from build123d import *

# Parameters (mm, degrees)
F2_R     = 5
F2_R_2   = 1.5
F3_DEPTH = 7.001
F4_D     = 2.5
F4_DEPTH = 3.2
F4_TIP   = 0.7510757738
F2_R_3   = 1.2
F5_DEPTH = 3.2


with BuildPart() as f1:
    # F0 (on Front) → F1 (revolve)
    with BuildSketch(Plane.XZ):
        Polygon((8.25, 7), (0, 7), (0, 0), (8.25, 0), (8.25, 0.9163741209), (7.85, 0.9163741209), (7.85, 1.9445925065), (8.25, 1.9445925065), (8.25, 3.9838924357), (7.85, 3.9838924357), (7.85, 5.2177544985), (8.25, 5.2177544985), align=None)
    revolve(axis=Axis((0, 0, 3.5), (0, 0, 1)))

    # F2 (on Top) → F3 (cut, through all)
    with BuildSketch(Plane.XY):
        with Locations((2.75, 0)):
            Circle(F2_R)
        with Locations((-4.75, 0)):
            Circle(F2_R_2)
    extrude(amount=F3_DEPTH, mode=Mode.SUBTRACT)

    # F4
    with Locations(Plane(origin=(0, 0, 0), x_dir=(1, 0, 0), z_dir=(0, 0, -1))):
        with Locations((0, 5.75), (0, -5.75)):
            Hole(F4_D / 2, depth=F4_DEPTH)
            with Locations((0, 0, -(F4_DEPTH + F4_TIP / 2))):  # 118° drill point
                Cone(0, F4_D / 2, F4_TIP, mode=Mode.SUBTRACT)

    # F2 (on Top) → F5 (cut)
    with BuildSketch(Plane.XY):
        with Locations((0, 5.75)):
            Circle(F2_R_3)
        with Locations((0, -5.75)):
            Circle(F2_R_3)
    extrude(amount=F5_DEPTH, mode=Mode.SUBTRACT)


solid = f1.part
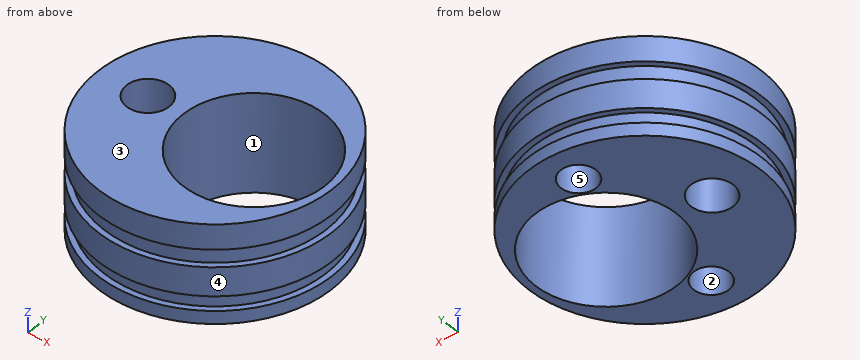
Source: CAD feature listing. Evaluate the final solid. Frame: model axes, mm. Face numbers are marked on the shaded views. A direction names the side the tool comes from. Give positions to 0.01 mm unless a question says otherwise; leave off trailing zeros. Write each loop counter-clockwise with the first axis right and the second up, starting at its lowest first coordinate (ties: lowest second). Pieces come first, ordered by that corner, then holes. Notation, with made-up numbers: M 78.5,72 L 114.5,72 A32 ccw 114.5,102 Z; hole C 60,-4.5 d2. An arc over 180 degrees is marked long. Return JSON: item names as keys, results as strings. Group by question number.
1) Set-up query: the marked faces 1 and 2. Return all of +Z, -Z, +X, -X, +Y, -Y with unobstructed straight access to the full face (end or side cutting, diameter ignored); none if empty.
2) Cut plane C-C, the plane y = 3.5. Output: boundary loops of the cut face in (x, z), then the cut area to 3 significant figures.
3) Draft query along Y for the marked faces 3, 4 and 5. Return one class per face: released by +Y, released by -Y, zero draft, split by the parting line, or undercut.
4) Cut plane D-D, the plane y = 1.25. Output: boundary loops of the cut face in (x, z).
5) Cut plane A-A, the plane x = 1.75. Output: boundary loops of the cut face in (y, z), then the cut area to 3 significant figures.
6) First-contact query: pin 1 Ø2 at (y, z) = (-5, 1) entering from +X; pin 2 Ø1.5 at (x, y) = (0, 5.75) entering from -Z. Flat tips, straight axial feed; report the tip coordinate or a pass-through.
7) Cut plane B-B, the plane z = 2.25. Output: boundary loops of the cut face in (x, y), then the cut area to 3 significant figures.
8) Ray query, L1, parallel to Y at x = 0.75, z = 1.5; L2, parallel to Y at x = 0, z = 0.7; L3, parallel to Y at x = -1.25, z = 5.25. Return the intervals inside material, ascending.
Data:
{
 "1": {"face 1": "+Z, -Z", "face 2": "-Z"},
 "2": {"outline": "M -7.47,0 L -0.82,0 L -0.82,7 L -7.47,7 L -7.47,5.22 L -7.03,5.22 L -7.03,3.98 L -7.47,3.98 L -7.47,1.94 L -7.03,1.94 L -7.03,0.92 L -7.47,0.92 Z; M 6.32,0 L 7.47,0 L 7.47,0.92 L 7.03,0.92 L 7.03,1.94 L 7.47,1.94 L 7.47,3.98 L 7.03,3.98 L 7.03,5.22 L 7.47,5.22 L 7.47,7 L 6.32,7 Z", "area": "52.6 mm²"},
 "3": {"face 3": "zero draft", "face 4": "split by the parting line", "face 5": "undercut"},
 "4": {"outline": "M -8.15,0 L -5.58,0 L -5.58,7 L -8.15,7 L -8.15,5.22 L -7.75,5.22 L -7.75,3.98 L -8.15,3.98 L -8.15,1.94 L -7.75,1.94 L -7.75,0.92 L -8.15,0.92 Z; M -3.92,0 L -2.09,0 L -2.09,7 L -3.92,7 Z; M 7.59,0 L 8.15,0 L 8.15,0.92 L 7.75,0.92 L 7.75,1.94 L 8.15,1.94 L 8.15,3.98 L 7.75,3.98 L 7.75,5.22 L 8.15,5.22 L 8.15,7 L 7.59,7 Z"},
 "5": {"outline": "M -8.06,0 L -4.9,0 L -4.9,7 L -8.06,7 L -8.06,5.22 L -7.65,5.22 L -7.65,3.98 L -8.06,3.98 L -8.06,1.94 L -7.65,1.94 L -7.65,0.92 L -8.06,0.92 Z; M 4.9,0 L 8.06,0 L 8.06,0.92 L 7.65,0.92 L 7.65,1.94 L 8.06,1.94 L 8.06,3.98 L 7.65,3.98 L 7.65,5.22 L 8.06,5.22 L 8.06,7 L 4.9,7 Z", "area": "42.4 mm²"},
 "6": {"pin 1": "stops at x = 7.21", "pin 2": "stops at z = 3.5"},
 "7": {"outline": "C 0,0 d16.5; hole C -4.75,0 d3; hole C 2.75,0 d10; hole C 0,-5.75 d2.5; hole C 0,5.75 d2.5", "area": "118 mm²"},
 "8": {"L1": "y = -7.81 to -6.75, -4.75 to -4.58, 4.58 to 4.75, 6.75 to 7.81", "L2": "y = -8.25 to -7, -4.5 to -4.18, 4.18 to 4.5, 7 to 8.25", "L3": "y = -8.15 to -3, 3 to 8.15"}
}
